Model file for the job. Use its own axes, mm. A direction names the side the tool comes from. Round coordinates to 2 decimals unless told otherwise and drop trailing zeros. Write each loop counter-clockwise with the first axis right and the second up, starting at its lowest first coordinate (ties: lowest second). Pieces come first, ordered by that corner, then holes.
```python
from build123d import *

# Parameters (mm, degrees)
SKETCH1_W           = 4.7625
SKETCH1_H           = 3.175
SKETCH1_W_2         = 3.175
SKETCH1_H_2         = 6.35
BOSS_EXTRUDE1_DEPTH = 3.175


with BuildPart() as part:
    # Sketch1 → Boss-Extrude1 (new body)
    with BuildSketch(Plane(origin=(0, 0, 0), x_dir=(1, 0, 0), z_dir=(0, 1, 0))):
        Polygon((-41.275, -12.7), (-41.275, 12.7), (-44.45, 12.7), (-44.45, 25.4), (-41.275, 25.4), (41.275, 25.4), (44.45, 25.4), (44.45, 12.7), (41.275, 12.7), (41.275, -12.7), (44.45, -12.7), (44.45, -25.4), (41.275, -25.4), (-41.275, -25.4), (-44.45, -25.4), (-44.45, -12.7), align=None)
        with Locations((0, 11.303)):
            Rectangle(SKETCH1_W, SKETCH1_H, mode=Mode.SUBTRACT)
        with Locations((0, -12.8905)):
            Rectangle(SKETCH1_W_2, SKETCH1_H_2, mode=Mode.SUBTRACT)
    extrude(amount=BOSS_EXTRUDE1_DEPTH)


solid = part.part
```
1) Cut at B-B on y = 2.1. Give the number of separate pieces and of enclosed holes in the cut face, and give its area (3 significant figures).
2) Cut at C-C on z = -1.5. List the corners of the cut face in (x, y) (3 decimals).
3) Wall check: probe 1 along X at (y, z) = (0.3, -11.5) (3 decimals); probe 2 along X at (y, z) = (1, 3) (3 decimals). Give the ranges that are in metal, low to high.
4) Flat gauge pins, fed straight in: pin 1 Ø1.6 at (y, z) = (1.5, -11.5) entering from -X (3 decimals); pin 2 Ø1 at (y, z) = (1.5, -11) entering from +X (3 decimals). Where does each tip first touch, or does it go through?
5) Which spindle directions (+Z, -Z, +X, -X, +Y, -Y) get a long thin tool onto all of the face, cutting with end or side? Do faces 1 (the face through (-41.275, 2, 0)), 2 (the face through (41.275, 2, 0)), 3 (the face through (-2.381, 2, -11)). Say none if no direction does.
6) Cut at A-A on z = -11. List the corners of the cut face in (x, y) (3 decimals), and give its area (3 significant figures).
Result sheet:
1. separate pieces: 1
1. enclosed holes: 2
1. area: 4,320 mm2
2. outline: (-41.275, 0) - (41.275, 0) - (41.275, 3.175) - (-41.275, 3.175) - close
3. probe 1: x = -41.275 to -2.381, 2.381 to 41.275
3. probe 2: x = -41.275 to 41.275
4. pin 1: stops at x = -41.275
4. pin 2: stops at x = 41.275
5. face 1: -X, +Y, -Y
5. face 2: +X, +Y, -Y
5. face 3: +Y, -Y
6. outline: (-41.275, 0) - (-2.381, 0) - (-2.381, 3.175) - (-41.275, 3.175) - close; (2.381, 0) - (41.275, 0) - (41.275, 3.175) - (2.381, 3.175) - close
6. area: 247 mm2
